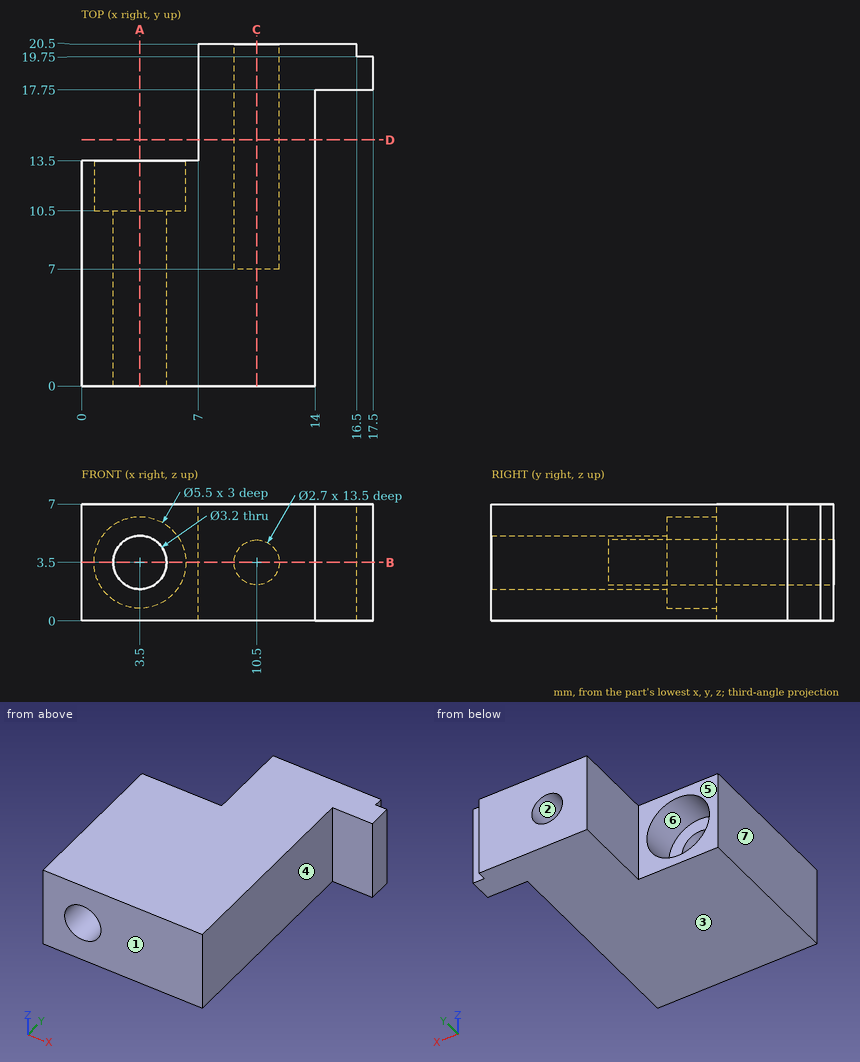
Input: dimensioned drawing with shaded views. Units: mm. Origin: part minimum x, y, z. A direction names the side the tool comes from. Coordinates: 2 decimals unless noted, no trailing zeros. Order: outer loops, then holes, each group sorted by start corner. A loop starts at its lowest first (then second) coordinate and runs counter-clockwise, first axis right, second up. Notation, with made-up numbers: (88.25, 56) - (102.25, 56) arc R16 cw to (102.25, 80) - close; hole circle Ø7 at (61.25, 56.5). An arc over 180 degrees is marked (long way). Put each result on its own line as item: value.
1. Line query: line 1 along X through (y, z) = (10.25, 3.5); line 2 along X through (y, z) = (6.5, 3.5); line 3 along X through (y, z) = (14.5, 3.5). Output: solid intervals per line, ascending.
Report:
line 1: x = 0 to 1.9, 5.1 to 9.15, 11.85 to 14
line 2: x = 0 to 1.9, 5.1 to 14
line 3: x = 7 to 9.15, 11.85 to 14
2. Contact query for flat-ended pins moving along their axis: pin 1 Ø2 at (y, z) = (17, 4) entering from -X; pin 2 Ø3 at (x, y) = (14.5, 15.5) entering from +Z; pin 3 Ø1.5 at (x, z) = (3.5, 2.5) entering from +Y; pin 4 Ø3.5 at (y, z) = (6.5, 3.5) entering from +X. Output: stop coordinate, or through.
Report:
pin 1: stops at x = 7
pin 2: stops at z = 7
pin 3: stops at y = 10.5
pin 4: stops at x = 14
3. Cut plane C-C on x = 10.5. Return the cut outline in (y, z).
Report:
outline: (0, 0) - (20.5, 0) - (20.5, 2.15) - (7, 2.15) - (7, 4.85) - (20.5, 4.85) - (20.5, 7) - (0, 7) - close
4. Cut plane B-B on z = 3.5. Return the cut outline in (x, y).
Report:
outline: (0, 0) - (1.9, 0) - (1.9, 10.5) - (0.75, 10.5) - (0.75, 13.5) - (0, 13.5) - close; (5.1, 0) - (14, 0) - (14, 17.75) - (17.5, 17.75) - (17.5, 19.75) - (16.5, 19.75) - (16.5, 20.5) - (11.85, 20.5) - (11.85, 7) - (9.15, 7) - (9.15, 20.5) - (7, 20.5) - (7, 13.5) - (6.25, 13.5) - (6.25, 10.5) - (5.1, 10.5) - close
5. Cut plane D-D on y = 14.75. Return the cut outline in (x, z).
Report:
outline: (7, 0) - (14, 0) - (14, 7) - (7, 7) - close; hole circle Ø2.7 at (10.5, 3.5)
6. Reachability of the marked faces 4, 5, 6 and 7 from +Z, -Z, +X, -X, +Y, -Y: full face, straight path, thin tool, end or side. Return the list, or none.
Report:
face 4: +Z, -Z, +X, -Y
face 5: +Z, -Z, -X, +Y
face 6: +Y
face 7: +Z, -Z, -X, +Y, -Y
7. Cut plane A-A on x = 3.5. Return the cut outline in (y, z), then the cut area to 3 significant figures.
Report:
outline: (0, 0) - (13.5, 0) - (13.5, 0.75) - (10.5, 0.75) - (10.5, 1.9) - (0, 1.9) - close; (0, 5.1) - (10.5, 5.1) - (10.5, 6.25) - (13.5, 6.25) - (13.5, 7) - (0, 7) - close
area: 44.4 mm2
8. Draft query along Z for the marked faces 1, 2 and 3. Return one class per face: pulls with the +Z half, pulls with the -Z half, needs draft (parallel to the pull), parting line crosses it, or undercut.
Report:
face 1: needs draft
face 2: undercut
face 3: pulls with the -Z half
